Geometry: final body of the model. Coordinates: model frame, mm. A direction names the side the tool comes from. Give positions to 0.01 mm unless a question says otherwise; leave off trailing zeros. Loops run counter-clockwise (first coordinate to the right, second up) from the corner with the lowest first, then second, coordinate; pieces in that order, holes last.
Autodesk Inventor part; units mm, degrees
ref_plane "作業平面1" through (16, -16, 100) normal (1, 0, 0) x (0, 0, -1)
ref_plane "YZ Plane" through (0, 0, 0) normal (1, 0, 0) x (0, 1, 0)
ref_plane "XZ Plane" through (0, 0, 0) normal (0, 1, 0) x (-1, 0, 0)
sketch "スケッチ1" plane through (0, 0, 0) normal (0, 0, 1) x (1, 0, 0)
  line L0 (-16, -16) -> (16, -16)
  line L1 (16, -16) -> (16, 16)
  line L2 (16, 16) -> (-16, 16)
  line L3 (-16, 16) -> (-16, -16)
  line L4 (-16, -16) -> (16, 16) construction
  line L5 (16, -16) -> (-16, 16) construction
  line L6 (-14.4, 14.4) -> (14.4, 14.4)
  line L7 (14.4, 14.4) -> (14.4, -14.4)
  line L8 (14.4, -14.4) -> (-14.4, -14.4)
  line L9 (-14.4, -14.4) -> (-14.4, 14.4)
  point P0 (0, 0)
  dimension "d0" = 32
  dimension "d1" = 32
  dimension "d2" = 1.6
extrude "押し出し1" add sketch "スケッチ1" along normal mid plane 200
ref_plane "作業平面1" through (16, -16, 100) normal (1, 0, 0) x (0, 0, -1)
sketch "スケッチ6" plane through (16, -16, 100) normal (1, 0, 0) x (0, 0, -1)
  line L0 (0, 0) -> (0, 32)
  line L1 (200, 32) -> (200, 0)
  point P0 (100, 16)
  point P1 (34.25, 16)
  point P2 (165.75, 16)
  dimension "d20" = 34.25
  dimension "d21" = 34.25
hole "穴2" at (16, 0, 65.75) at (16, 0, -65.75) direction (-1, 0, 0) diameter 14 end through all
properties part number "Pipe横"
Q1. Section query B-B, the plane x = 10. Return loops of the section in (y, z).
Q2. Section query C-C, the plane y = 0. Return loops of the section in (x, z), and give its area (3 significant figures).
Q3. Section query A-A, the plane z = -65.75. Return loops of the section in (x, y), and give its area (3 significant figures).
Q4. Reachability of faces 4 (the face through (15.189, -2.103, -72.427)), 5 (the face through (14.4, 0, -1)) from +Z, -Z, +X, -X, +Y, -Y: full face, straight path, thin tool, end or side. Return the list, or none.
Q5. Pin query (flat end, axial travel): pin 1 Ø11 at (y, z) = (0, 65.75) entering from -X (3 decimals). Return the tip coordinate at first contact, or that it passes through.
Q6. Material intervals for probe 1 along Z at (x, y) = (15.2, 0); probe 2 along X at (y, z) = (-12, -54), sorted ascending.
Q7. Mould query, pull axis Z, two halves, no side actions, for faces 1 (the face through (-15.211, 4.259, 71.305)), 2 (the face through (0, -16, -1)), 3 (the face through (-1, -15, 100)). Classes: +Z half, -Z half, draft (parallel to the pull), parting line (faces both ways), or undercut.
Resolved:
1. outline: (-16, -100) - (-14.4, -100) - (-14.4, 100) - (-16, 100) - close; (14.4, -100) - (16, -100) - (16, 100) - (14.4, 100) - close
2. outline: (-16, -100) - (-14.4, -100) - (-14.4, -72.75) - (-16, -72.75) - close; (-16, -58.75) - (-14.4, -58.75) - (-14.4, 58.75) - (-16, 58.75) - close; (-16, 72.75) - (-14.4, 72.75) - (-14.4, 100) - (-16, 100) - close; (14.4, -100) - (16, -100) - (16, -72.75) - (14.4, -72.75) - close; (14.4, -58.75) - (16, -58.75) - (16, 58.75) - (14.4, 58.75) - close; (14.4, 72.75) - (16, 72.75) - (16, 100) - (14.4, 100) - close
2. area: 550 mm2
3. outline: (-16, -16) - (16, -16) - (16, -7) - (14.4, -7) - (14.4, -14.4) - (-14.4, -14.4) - (-14.4, -7) - (-16, -7) - close; (-16, 7) - (-14.4, 7) - (-14.4, 14.4) - (14.4, 14.4) - (14.4, 7) - (16, 7) - (16, 16) - (-16, 16) - close
3. area: 150 mm2
4. face 4: +X, -X
4. face 5: +Z, -Z
5. pin 1: passes through
6. probe 1: z = -100 to -72.75, -58.75 to 58.75, 72.75 to 100
6. probe 2: x = -16 to -14.4, 14.4 to 16
7. face 1: undercut
7. face 2: draft
7. face 3: +Z half
